```python
from build123d import *

# Parameters (mm, degrees)
SKETCH1_W           = 7
SKETCH1_H           = 7
BOSS_EXTRUDE1_DEPTH = 1.5
SKETCH2_W           = 1.47
SKETCH2_H           = 1.47
BOSS_EXTRUDE2_DEPTH = 0.5
SKETCH3_W           = 1.02
SKETCH3_H           = 1.02
BOSS_EXTRUDE3_DEPTH = 3.94
SKETCH4_R           = 3.25
SKETCH4_R_2         = 1.6
BOSS_EXTRUDE4_DEPTH = 7.06
CHAMFER1_SIZE       = 0.125
SKETCH7_R           = 0.48
BOSS_EXTRUDE5_DEPTH = 4.44
CHAMFER2_SIZE       = 0.25


with BuildPart() as part:
    # Sketch1 → Boss-Extrude1 (new body)
    with BuildSketch(Plane(origin=(0, 0, 0), x_dir=(1, 0, 0), z_dir=(0, 1, 0))):
        Rectangle(SKETCH1_W, SKETCH1_H)
    extrude(amount=BOSS_EXTRUDE1_DEPTH)

    # Sketch2 → Boss-Extrude2 (add)
    with BuildSketch(Plane(origin=(0, 1.5, 0), x_dir=(1, 0, 0), z_dir=(0, 1, 0))):
        with Locations((-2.765, 2.765)):
            Rectangle(SKETCH2_W, SKETCH2_H)
        with Locations((2.765, 2.765)):
            Rectangle(SKETCH2_W, SKETCH2_H)
        with Locations((2.765, -2.765)):
            Rectangle(SKETCH2_W, SKETCH2_H)
        with Locations((-2.765, -2.765)):
            Rectangle(SKETCH2_W, SKETCH2_H)
    extrude(amount=BOSS_EXTRUDE2_DEPTH)

    # Sketch3 → Boss-Extrude3 (add)
    with BuildSketch(Plane(origin=(0, 2, 0), x_dir=(1, 0, 0), z_dir=(0, 1, 0))):
        with Locations((-2.54, -2.54)):
            Rectangle(SKETCH3_W, SKETCH3_H)
        with Locations((2.54, -2.54)):
            Rectangle(SKETCH3_W, SKETCH3_H)
        with Locations((2.54, 2.54)):
            Rectangle(SKETCH3_W, SKETCH3_H)
        with Locations((-2.54, 2.54)):
            Rectangle(SKETCH3_W, SKETCH3_H)
    extrude(amount=BOSS_EXTRUDE3_DEPTH)

    # Sketch4 → Boss-Extrude4 (add)
    with BuildSketch(Plane.XZ):
        with Locations(Location((0, 0, 0), (0, 0, 270))):
            Circle(SKETCH4_R)
        with Locations(Location((0, 0, 0), (0, 0, 270))):
            Circle(SKETCH4_R_2, mode=Mode.SUBTRACT)
    extrude(amount=BOSS_EXTRUDE4_DEPTH)

    # Chamfer1
    chamfer1_edges = [part.edges().sort_by_distance(p)[0] for p in [
        (0, -7.06, 1.6),
        (0, -7.06, 3.25),
    ]]
    chamfer(chamfer1_edges, length=CHAMFER1_SIZE)

    # Sketch5 → Cut-Revolve1 (revolve, cut)
    with BuildSketch(Plane.XY, mode=Mode.PRIVATE) as cut_revolve1_sk:
        Polygon((-3.25, -1.4675), (-3.125, -1.5925), (-3.125, -5.3425), (-3.25, -5.4675), align=None)
        Polygon((-3.25, 0), (-3.125, 0), (-3.25, -0.125), align=None)
    revolve(cut_revolve1_sk.sketch.rotate(Axis((0, -6.81, 0), (0, 1, 0)), 270), axis=Axis((0, -6.81, 0), (0, 1, 0)), mode=Mode.SUBTRACT)

    # Sketch7 → Boss-Extrude5 (add)
    with BuildSketch(Plane(origin=(0, 1.5, 0), x_dir=(1, 0, 0), z_dir=(0, 1, 0))):
        with Locations(Location((0, 0, 0), (0, 0, 90))):
            Circle(SKETCH7_R)
    extrude(amount=BOSS_EXTRUDE5_DEPTH)

    # Chamfer2
    chamfer2_edges = [part.edges().sort_by_distance(p)[0] for p in [
        (0, 5.94, 0.48),
    ]]
    chamfer(chamfer2_edges, length=CHAMFER2_SIZE)


solid = part.part
```
CAD build for the part. Positions are in the model's coordinates, mm. A direction names the side the tool comes from. Give positions to 0.01 mm unless a question says otherwise; leave off trailing zeros. Order: outer loops, then holes, each group sorted by start corner. A loop starts at its lowest first (then second) coordinate and runs counter-clockwise, first axis right, second up. Notation, with made-up numbers: M 74,78 L 111,78 A20 ccw 111,112 Z; hole C 88,7 d3. An arc over 180 degrees is marked long. Put each result on its own line as item: value. Start each with the question number.
(1) Which spindle directions (+Z, -Z, +X, -X, +Y, -Y) get a long thin tool onto all of the face, cutting with end or side? Do faces 1 (the flat face through (2.5, 3.9, -3.05)), 2 (the flat face through (2.5, 3.9, 3.05)), 3 (the cylindrical face through (-0.94, -3.49, -2.98)), 4 (the flat face through (-3.05, 3.9, 2.5)), 5 (the flat face through (-2.6, 3.7, -2.03)). Say none if no direction does.
(2) Flat gauge pins, fed straight in: pin 1 Ø0.5 at (y, z) = (4.5, 3) entering from +X; pin 2 Ø1.1 at (x, y) = (2.5, 3) entering from +Z; pin 3 Ø1.2 at (x, y) = (2.5, 3) entering from -Z. Where does each tip first touch, or does it go through?
(3) Drill centre lines: line 1 along X through (y, z) = (-4, 0) (3 decimals); line 2 along Z through (x, y) = (2.25, 5). Where is each one in solid material? Low to high.
(4) Mould opens along Z. For faces 6 (the cylindrical face through (-0.97, -3.42, 1.27)), 7 (the cylindrical face through (-1.978, -0.787, 2.579)), 8 (the flat face through (-3.5, 1, 0)) say: +Z half, -Z half, draft (parallel to the pull), parting line (faces both ways), or undercut.
(5) Saw through at C-C, the plane y = -4.5. Write the cut outline in (x, z) (3 decimals).
Check result:
1. face 1: -Z, +X, -X, +Y
1. face 2: +Z, +X, -X, +Y
1. face 3: none
1. face 4: +Z, -Z, -X, +Y
1. face 5: +X, -X, +Y
2. pin 1: stops at x = 3.05
2. pin 2: stops at z = 3.05
2. pin 3: stops at z = -3.05
3. line 1: x = -3.125 to -1.6, 1.6 to 3.125
3. line 2: z = -3.05 to -2.03, 2.03 to 3.05
4. face 6: undercut
4. face 7: parting line
4. face 8: draft
5. outline: C 0,0 d6.25; hole C 0,0 d3.2
